Input: part model. Units: mm. Frame: model coordinates. Round coordinates to 2 decimals unless told otherwise and drop trailing zeros. Loops run counter-clockwise (first coordinate to the right, second up) from the corner with the lowest first, then second, coordinate; pieces in that order, holes last. Notation, with made-up numbers: (41.25, -34) - (58.25, -34) arc R26 ccw to (58.25, -1) - close; hole circle Ø3 at (2.25, -12.75). An arc over 180 degrees is marked (long way). Write each question's results on one line, items separated by ' | '.
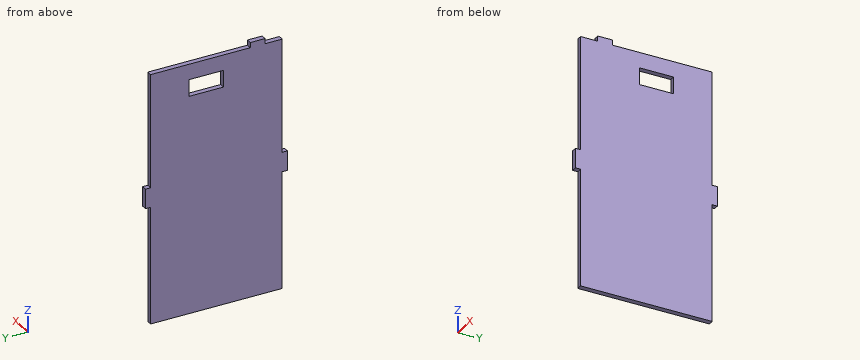
from build123d import *

# Parameters (mm, degrees)
SKETCH1_W           = 38.1
SKETCH1_H           = 40.325
BOSS_EXTRUDE1_DEPTH = 3.175
SKETCH3_W           = 3.175
SKETCH3_H           = 10.49
SKETCH3_H_2         = 20.695
CUT_EXTRUDE2_DEPTH  = 4.175
SKETCH5_W           = 3.175
SKETCH5_H           = 12
BOSS_EXTRUDE2_DEPTH = 3.175
SKETCH7_W           = 3.175
SKETCH7_H           = 80.65
BOSS_EXTRUDE3_DEPTH = 63
SKETCH8_W           = 3.175
SKETCH8_H           = 80.65
BOSS_EXTRUDE4_DEPTH = 55.929385
SKETCH9_W           = 3.175
SKETCH9_H           = 9.082720128
BOSS_EXTRUDE5_DEPTH = 3.18
SKETCH10_W          = 10.316938
SKETCH10_H          = 21.036408148
CUT_EXTRUDE3_DEPTH  = 3.18


with BuildPart() as part:
    # Sketch1 → Boss-Extrude1 (new body)
    with BuildSketch(Plane(origin=(0, 0, 0), x_dir=(0, 0, -1), z_dir=(1, 0, 0))):
        with Locations((-19.05, 20.1625)):
            Rectangle(SKETCH1_W, SKETCH1_H)
    boss_extrude1 = extrude(amount=BOSS_EXTRUDE1_DEPTH)

    # Sketch3 → Cut-Extrude2 (cut, through all)
    with BuildSketch(Plane(origin=(3.175, 0, 0), x_dir=(0, 0, -1), z_dir=(1, 0, 0))):
        with Locations((-36.5125, 35.08)):
            Rectangle(SKETCH3_W, SKETCH3_H)
        with Locations((-36.5125, 10.3475)):
            Rectangle(SKETCH3_W, SKETCH3_H_2)
    cut_extrude2 = extrude(amount=-CUT_EXTRUDE2_DEPTH, mode=Mode.SUBTRACT)

    # Sketch5 → Boss-Extrude2 (add)
    with BuildSketch(Plane(origin=(0, 0, 0), x_dir=(-1, 0, 0), z_dir=(0, -1, 0))):
        with Locations((-1.5875, -15.025)):
            Rectangle(SKETCH5_W, SKETCH5_H)
    boss_extrude2 = extrude(amount=BOSS_EXTRUDE2_DEPTH)

    # Mirror1: Boss-Extrude1, Cut-Extrude2, Boss-Extrude2 across plane
    add(boss_extrude1.mirror(Plane(origin=(3.175, 40.325, 0), x_dir=(0, 0, 1), z_dir=(0, -1, 0))))
    add(cut_extrude2.mirror(Plane(origin=(3.175, 40.325, 0), x_dir=(0, 0, 1), z_dir=(0, -1, 0))), mode=Mode.SUBTRACT)
    add(boss_extrude2.mirror(Plane(origin=(3.175, 40.325, 0), x_dir=(0, 0, 1), z_dir=(0, -1, 0))))

    # Sketch7 → Boss-Extrude3 (add)
    with BuildSketch(Plane(origin=(0, 0, 0), x_dir=(-1, 0, 0), z_dir=(0, 0, -1))):
        with Locations((-1.5875, 40.325)):
            Rectangle(SKETCH7_W, SKETCH7_H)
    extrude(amount=BOSS_EXTRUDE3_DEPTH)

    # Sketch8 → Boss-Extrude4 (add)
    with BuildSketch(Plane.XY.offset(34.925)):
        with Locations((1.5875, 40.325)):
            Rectangle(SKETCH8_W, SKETCH8_H)
    extrude(amount=BOSS_EXTRUDE4_DEPTH)

    # Sketch9 → Boss-Extrude5 (add)
    with BuildSketch(Plane.XY.offset(90.85438473)):
        with Locations((1.5875, 15.031360064)):
            Rectangle(SKETCH9_W, SKETCH9_H)
    extrude(amount=BOSS_EXTRUDE5_DEPTH)

    # Sketch10 → Cut-Extrude3 (cut)
    with BuildSketch(Plane(origin=(3.175, 0, 0), x_dir=(0, 0, -1), z_dir=(1, 0, 0))):
        with Locations((-76.199393077, 46.454229061)):
            Rectangle(SKETCH10_W, SKETCH10_H)
    extrude(amount=-CUT_EXTRUDE3_DEPTH, mode=Mode.SUBTRACT)


solid = part.part
1. Section query A-A, the plane y = 39. Output: boundary loops of the cut face in (x, z) (3 decimals).
Answer:
outline: (0, -63) - (3.175, -63) - (3.175, 71.041) - (0, 71.041) - close; (0, 81.358) - (3.175, 81.358) - (3.175, 90.854) - (0, 90.854) - close
2. Section query B-B, the plane x = 2.4. Output: boundary loops of the cut face in (y, z) (3 decimals).
Answer:
outline: (-3.175, 9.025) - (0, 9.025) - (0, -63) - (80.65, -63) - (80.65, 9.025) - (83.825, 9.025) - (83.825, 21.025) - (80.65, 21.025) - (80.65, 90.854) - (19.573, 90.854) - (19.573, 94.034) - (10.49, 94.034) - (10.49, 90.854) - (0, 90.854) - (0, 21.025) - (-3.175, 21.025) - close; hole (35.936, 71.041) - (56.972, 71.041) - (56.972, 81.358) - (35.936, 81.358) - close
3. Line query: line 1 (Z direction, x = 1.8, y = 37.5); line 2 (Z direction, x = 2.8, y = 24.5); line 3 (Y direction, x = 2.95, z = -48.5). Output: solid intervals per line, ascending. Write a range as [from, to].
Answer:
line 1: [-63, 71.04], [81.36, 90.85] | line 2: [-63, 90.85] | line 3: [0, 80.65]
4. Section query C-C, the plane z = 79. Output: boundary loops of the cut face in (x, y) (3 decimals), plus the area to 3 significant figures.
Answer:
outline: (0, 0) - (3.175, 0) - (3.175, 35.936) - (0, 35.936) - close; (0, 56.972) - (3.175, 56.972) - (3.175, 80.65) - (0, 80.65) - close | area: 189 mm^2
5. Contact query for flat-ended pins moving along their axis: pin 1 (1.6 mm diameter, centred on x = 1, y = 82, fed in from -Z) (3 decimals); pin 2 (1.6 mm diameter, centred on x = 1.5, z = 92.5, fed in from -Y); pin 3 (1.6 mm diameter, centred on x = 1.5, z = 92, fed in from +Y). Output: stop coordinate, or through.
Answer:
pin 1: z = 9.025 | pin 2: y = 10.49 | pin 3: y = 19.57
6. Section query D-D, the plane y = 27.5. Output: boundary loops of the cut face in (x, z) (3 decimals).
Answer:
outline: (0, -63) - (3.175, -63) - (3.175, 90.854) - (0, 90.854) - close
